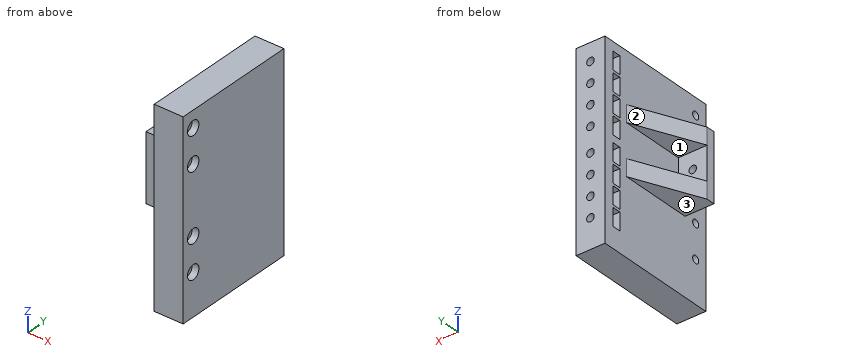
```python
from build123d import *
from OCP.BRepFilletAPI import BRepFilletAPI_MakeChamfer

# Parameters (mm, degrees)
SKETCH1_W                               = 115
SKETCH1_H                               = 75
BOSS_EXTRUDE1_DEPTH                     = 17.272
M4_CLEARANCE_HOLE1_AT_2_COUNT           = 2
M4_CLEARANCE_HOLE1_AT_2_PITCH           = 50.8
SKETCH5_W                               = 10.5
SKETCH5_H                               = 5
CUT_EXTRUDE1_DEPTH                      = 14.08
LPATTERN1_COUNT                         = 2
LPATTERN1_PITCH                         = 12
LPATTERN1_COL_COUNT                     = 3
LPATTERN1_COL_PITCH                     = 12
CBORE_FOR_M5_HEX_HEAD_BOLT1_D           = 4.5
CBORE_FOR_M5_HEX_HEAD_BOLT1_CBORE_D     = 8.5
CBORE_FOR_M5_HEX_HEAD_BOLT1_CBORE_DEPTH = 4
BOSS_EXTRUDE3_DEPTH                     = 17.228
CHAMFER2_SIZE                           = 17.228
CHAMFER2_SIZE_2                         = 38.6
M4_CLEARANCE_HOLE3_D                    = 4.5


with BuildPart() as part:
    # Sketch1 → Boss-Extrude1 (new body)
    with BuildSketch(Plane(origin=(0, 0, 0), x_dir=(0, 0, -1), z_dir=(1, 0, 0))):
        Rectangle(SKETCH1_W, SKETCH1_H)
    extrude(amount=BOSS_EXTRUDE1_DEPTH)

    # Sketch4 → M4 Clearance Hole1 (revolve, cut)
    with BuildSketch(Plane(origin=(8.692, 37.5, 22.9), x_dir=(0, 0, 1), z_dir=(1, 0, 0))):
        Polygon((0, 0), (0, 7.351936393), (2.25, 6), (2.25, 0), align=None)
    m4_clearance_hole1 = revolve(axis=Axis((8.692, 43.85, 22.9), (0, -1, 0)), mode=Mode.SUBTRACT)

    # M4 Clearance Hole1 at 2: M4 Clearance Hole1 ×2
    with Locations(*[(0, 0, -i * M4_CLEARANCE_HOLE1_AT_2_PITCH) for i in range(1, M4_CLEARANCE_HOLE1_AT_2_COUNT)]):
        add(m4_clearance_hole1, mode=Mode.SUBTRACT)

    # Sketch5 → Cut-Extrude1 (cut)
    with BuildSketch(Plane.ZY):
        with Locations((-27.9, 29)):
            Rectangle(SKETCH5_W, SKETCH5_H)
        with Locations((22.9, 29)):
            Rectangle(SKETCH5_W, SKETCH5_H)
    cut_extrude1 = extrude(amount=-CUT_EXTRUDE1_DEPTH, mode=Mode.SUBTRACT)

    # LPattern1: M4 Clearance Hole1, Cut-Extrude1 ×2
    with Locations(*[(0, 0, -i * LPATTERN1_PITCH) for i in range(1, LPATTERN1_COUNT)]):
        add(m4_clearance_hole1, mode=Mode.SUBTRACT)
        add(cut_extrude1, mode=Mode.SUBTRACT)

    # LPattern1 copy 1 sketch → LPattern1 copy 1 (revolve, cut)
    with BuildSketch(Plane(origin=(8.692, 37.5, -39.9), x_dir=(0, 0, 1), z_dir=(1, 0, 0))):
        Polygon((0, 0), (0, 7.351936393), (2.25, 6), (2.25, 0), align=None)
    revolve(axis=Axis((8.692, 43.85, -39.9), (0, -1, 0)), mode=Mode.SUBTRACT)

    # LPattern1 col: M4 Clearance Hole1, Cut-Extrude1 ×3
    with Locations(*[(0, 0, i * LPATTERN1_COL_PITCH) for i in range(1, LPATTERN1_COL_COUNT)]):
        add(m4_clearance_hole1, mode=Mode.SUBTRACT)
        add(cut_extrude1, mode=Mode.SUBTRACT)

    # LPattern1 col copy 1 sketch → LPattern1 col copy 1 (revolve, cut)
    with BuildSketch(Plane(origin=(8.692, 37.5, -15.9), x_dir=(0, 0, 1), z_dir=(1, 0, 0))):
        Polygon((0, 0), (0, 7.351936393), (2.25, 6), (2.25, 0), align=None)
    revolve(axis=Axis((8.692, 43.85, -15.9), (0, -1, 0)), mode=Mode.SUBTRACT)

    # LPattern1 col copy 2 sketch → LPattern1 col copy 2 (revolve, cut)
    with BuildSketch(Plane(origin=(8.692, 37.5, -3.9), x_dir=(0, 0, 1), z_dir=(1, 0, 0))):
        Polygon((0, 0), (0, 7.351936393), (2.25, 6), (2.25, 0), align=None)
    revolve(axis=Axis((8.692, 43.85, -3.9), (0, -1, 0)), mode=Mode.SUBTRACT)

    # CBORE for M5 Hex Head Bolt1 (through all)
    with Locations(Plane(origin=(17.272, 0, 0), x_dir=(0, 0, -1), z_dir=(1, 0, 0))):
        with Locations((32.5, -30), (12.5, -30), (-27.5, -30), (-47.5, -30)):
            CounterBoreHole(CBORE_FOR_M5_HEX_HEAD_BOLT1_D / 2, CBORE_FOR_M5_HEX_HEAD_BOLT1_CBORE_D / 2, CBORE_FOR_M5_HEX_HEAD_BOLT1_CBORE_DEPTH)

    # Sketch12 → Boss-Extrude3 (add)
    with BuildSketch(Plane.ZY):
        Polygon((-12.5, 21.5), (-12.5, -22.1), (27.5, -22.1), (27.5, 21.5), (17.5, 21.5), (17.5, -17.1), (-2.5, -17.1), (-2.5, 21.5), align=None)
    extrude(amount=BOSS_EXTRUDE3_DEPTH)

    # Chamfer2
    chamfer2_edges_1 = [part.edges().sort_by_distance(p)[0] for p in [
        (-17.228, 21.5, -7.5),
    ]]
    chamfer2_side_1 = [part.faces().sort_by_distance(p)[0] for p in [
        (-16.88344, 21.5, -7.5),
    ]]
    chamfer2_edges_2 = [part.edges().sort_by_distance(p)[0] for p in [
        (-17.228, 21.5, 22.5),
    ]]
    chamfer2_side_2 = [part.faces().sort_by_distance(p)[0] for p in [
        (-16.88344, 21.5, 22.5),
    ]]
    chamfer2 = BRepFilletAPI_MakeChamfer(part.part.solid().wrapped)
    for e in chamfer2_edges_1:
        chamfer2.Add(CHAMFER2_SIZE - 0.0001, CHAMFER2_SIZE_2 - 0.0001, e.wrapped, chamfer2_side_1[0].wrapped)
    for e in chamfer2_edges_2:
        chamfer2.Add(CHAMFER2_SIZE - 0.0001, CHAMFER2_SIZE_2 - 0.0001, e.wrapped, chamfer2_side_2[0].wrapped)
    add(Compound.cast(chamfer2.Shape()), mode=Mode.REPLACE)  # a hair under: the kernel refuses the full size

    # M4 Clearance Hole3 (through all)
    with Locations(Plane(origin=(0, -17.1, 0), x_dir=(1, 0, 0), z_dir=(0, 1, 0))):
        with Locations((-8.614, -7.5)):
            Hole(M4_CLEARANCE_HOLE3_D / 2)


solid = part.part
```
Here's how the part is built. I have some questions about the finished solid (model axes, mm). Face numbers are marked on the shaded views. A direction names the side the tool comes from. Round coordinates to 2 decimals unless told otherwise and drop trailing zeros. Loops run counter-clockwise (first coordinate to the right, second up) from the corner with the lowest first, then second, coordinate; pieces in that order, holes last.
1. If I drill on probe 1 along Y at (x, z) = (12.5, 35); probe 2 along Z at (x, y) = (-2, -13.5); probe 3 along X at (y, z) = (34.1, -15.9), over which ranges is the centre line in solid material (lowest first)?
Answers:
probe 1: y = -37.5 to 26.5, 31.5 to 37.5
probe 2: z = -12.5 to -2.5, 17.5 to 27.5
probe 3: x = 0 to 6.44, 10.94 to 17.27
2. Suppose I cut it at D-D, the plane x = -14. Please give me the cut outline in (y, z), and give its area (3 significant figures).
Answers:
outline: (-22.1, -12.5) - (-9.87, -12.5) - (-9.87, -2.5) - (-17.1, -2.5) - (-17.1, 17.5) - (-9.87, 17.5) - (-9.87, 27.5) - (-22.1, 27.5) - close
area: 345 mm2
3. Suppose I cut it at C-C, the plane y = 0. Please give me the cut outline in (x, z).
Answers:
outline: (-9.6, -12.5) - (0, -12.5) - (0, -57.5) - (17.27, -57.5) - (17.27, 57.5) - (0, 57.5) - (0, 27.5) - (-9.6, 27.5) - (-9.6, 17.5) - (0, 17.5) - (0, -2.5) - (-9.6, -2.5) - close
4. Suppose I cut it at A-A, the plane z = -39.9. Please give me the cut outline in (x, y), and give its area (3 significant figures).
Answers:
outline: (0, -37.5) - (17.27, -37.5) - (17.27, 37.5) - (10.94, 37.5) - (10.94, 31.5) - (14.08, 31.5) - (14.08, 26.5) - (0, 26.5) - close; (0, 31.5) - (6.44, 31.5) - (6.44, 37.5) - (0, 37.5) - close
area: 1,200 mm2
5. Suppose I cut it at B-B, the plane z = 46.9. Please give me the cut outline in (x, y).
Answers:
outline: (0, -37.5) - (17.27, -37.5) - (17.27, -34.21) - (13.27, -34.21) - (13.27, -32.17) - (0, -32.17) - close; (0, -27.83) - (13.27, -27.83) - (13.27, -25.79) - (17.27, -25.79) - (17.27, 37.5) - (10.94, 37.5) - (10.94, 31.5) - (14.08, 31.5) - (14.08, 26.5) - (0, 26.5) - close; (0, 31.5) - (6.44, 31.5) - (6.44, 37.5) - (0, 37.5) - close
6. Will these pins go through, and if not, where does the flat tip stop? pin 1 (4 mm diameter, centred on y = -24, z = -45, fed in from -X); pin 2 (5 mm diameter, centred on x = 7.5, z = 10, fed in from +Y); pin 3 (1.5 mm diameter, centred on y = 29.5, z = 12.5, fed in from -X); pin 4 (5 mm diameter, centred on y = -1, z = -13, fed in from -X).
Answers:
pin 1: stops at x = 0
pin 2: stops at y = 37.5
pin 3: stops at x = 14.08
pin 4: stops at x = -11.14
7. For the marked faces 1, 2 and 3, which set-ups out of +Z, -Z, +X, -X, +Y, -Y let a thin tool reach every point of the face, with its end or its side?
Answers:
face 1: -X, +Y
face 2: +Z, -Z, -X, +Y
face 3: -Z, -X, +Y, -Y
